```python
from build123d import *

# Parameters (mm, degrees)
SKETCH1_W                                     = 230
SKETCH1_H                                     = 123
SKETCH1_W_2                                   = 206
SKETCH1_H_2                                   = 99
BOSS_EXTRUDE1_DEPTH                           = 5
SKETCH2_W                                     = 230
SKETCH2_H                                     = 5
BOSS_EXTRUDE2_DEPTH                           = 6
BOSS_EXTRUDE3_DEPTH                           = 5
FILLET1_R                                     = 15
BOSS_EXTRUDE4_DEPTH                           = 4
FILLET2_R                                     = 5
FILLET3_R                                     = 3
CSK_FOR_4_FLAT_HEAD_MACHINE_SCREW1_AT_2_COUNT = 2
CSK_FOR_4_FLAT_HEAD_MACHINE_SCREW1_AT_2_PITCH = 30
CSK_FOR_4_FLAT_HEAD_MACHINE_SCREW1_AT_3_COUNT = 2
CSK_FOR_4_FLAT_HEAD_MACHINE_SCREW1_AT_3_PITCH = 225.008888713
CSK_FOR_4_FLAT_HEAD_MACHINE_SCREW1_AT_4_COUNT = 2
CSK_FOR_4_FLAT_HEAD_MACHINE_SCREW1_AT_4_PITCH = 223


with BuildPart() as part:
    # Sketch1 → Boss-Extrude1 (new body)
    with BuildSketch(Plane.XY):
        Rectangle(SKETCH1_W, SKETCH1_H)
        Rectangle(SKETCH1_W_2, SKETCH1_H_2, mode=Mode.SUBTRACT)
    extrude(amount=BOSS_EXTRUDE1_DEPTH)

    # Sketch2 → Boss-Extrude2 (add)
    with BuildSketch(Plane(origin=(0, 61.5, 0), x_dir=(1, 0, 0), z_dir=(0, 1, 0))):
        Polygon((-115, 10), (-115, 0), (115, 0), (115, 10), (115, 93), (105, 93), (105, 10), (-105, 10), (-105, 93), (-115, 93), align=None)
        with Locations((0, -2.5)):
            Rectangle(SKETCH2_W, SKETCH2_H)
    boss_extrude2 = extrude(amount=BOSS_EXTRUDE2_DEPTH)

    # Mirror1: Boss-Extrude2 across plane
    add(boss_extrude2.mirror(Plane.ZX))

    # Sketch3 → Boss-Extrude3 (add)
    with BuildSketch(Plane.ZY.offset(115)):
        Polygon((-93, 61.5), (0, 61.5), (0, -61.5), (-93, -61.5), (-93, -67.5), (5, -67.5), (5, 67.5), (-93, 67.5), align=None)
        Polygon((0, 61.5), (-25, 61.5), (-20, 55.5), (0, 31.5), align=None)
        Polygon((0, -61.5), (0, -31.5), (-20, -55.5), (-25, -61.5), align=None)
        Polygon((-20, 55.5), (-25, 61.5), (-93, 61.5), (-93, 55.5), align=None)
        Polygon((-25, -61.5), (-20, -55.5), (-93, -55.5), (-93, -61.5), align=None)
    boss_extrude3 = extrude(amount=BOSS_EXTRUDE3_DEPTH)

    # Mirror2: Boss-Extrude3 across plane
    add(boss_extrude3.mirror(Plane(origin=(0, 0, 0), x_dir=(0, 0, 1), z_dir=(1, 0, 0))))

    # Fillet1
    fillet1_edges = [part.edges().sort_by_distance(p)[0] for p in [
        (117.5, 55.5, -20),
        (117.5, -55.5, -20),
        (117.5, -31.5, 0),
        (117.5, 31.5, 0),
        (-103, -49.5, 2.5),
        (103, -49.5, 2.5),
        (103, 49.5, 2.5),
        (-103, 49.5, 2.5),
        (105, 64.5, -10),
        (-105, 64.5, -10),
        (-105, -64.5, -10),
        (105, -64.5, -10),
        (-117.5, 55.5, -20),
        (-117.5, 31.5, 0),
        (-117.5, -31.5, 0),
        (-117.5, -55.5, -20),
    ]]
    fillet(fillet1_edges, radius=FILLET1_R)

    # Sketch4 → Boss-Extrude4 (add, symmetric)
    with BuildSketch(Plane(origin=(0, 0, 0), x_dir=(1, 0, 0), z_dir=(0, 1, 0))):
        Polygon((-120, 96.464101615), (-120, 0), (-116.5, 0), (-116.5, 90), (-110.5, 93.464101615), (-110.5, 96.464101615), align=None)
    extrude(amount=BOSS_EXTRUDE4_DEPTH, both=True)

    # Fillet2
    fillet2_edges = [part.edges().sort_by_distance(p)[0] for p in [
        (-118.25, 4, 0),
        (-118.25, -4, 0),
    ]]
    fillet(fillet2_edges, radius=FILLET2_R)

    # Fillet3
    fillet3_edges = [part.edges().sort_by_distance(p)[0] for p in [
        (120, 61.5, -93),
        (120, -61.5, -93),
        (105, 64.5, -93),
        (-120, 0, -96.464101615),
        (-105, 64.5, -93),
        (-105, -64.5, -93),
        (105, -64.5, -93),
        (-120, -61.5, -93),
        (-120, 61.5, -93),
    ]]
    fillet(fillet3_edges, radius=FILLET3_R)

    # Sketch6 → CSK for #4 Flat Head Machine Screw1 (revolve, cut)
    with BuildSketch(Plane(origin=(111.5, 61.5, -68), x_dir=(0, 0, -1), z_dir=(1, 0, 0))):
        Polygon((0, 0), (0, 6), (1.63195, 6), (1.63195, 2.409835609), (2.857501397, 1), (2.857501397, 0), align=None)
    csk_for_4_flat_head_machine_screw1 = revolve(axis=Axis((111.5, 55.15, -68), (0, 1, 0)), mode=Mode.SUBTRACT)

    # CSK for #4 Flat Head Machine Screw1 at 2: CSK for #4 Flat Head Machine Screw1 ×2
    with Locations(*[(0, 0, i * CSK_FOR_4_FLAT_HEAD_MACHINE_SCREW1_AT_2_PITCH) for i in range(1, CSK_FOR_4_FLAT_HEAD_MACHINE_SCREW1_AT_2_COUNT)]):
        add(csk_for_4_flat_head_machine_screw1, mode=Mode.SUBTRACT)

    # CSK for #4 Flat Head Machine Screw1 at 3: CSK for #4 Flat Head Machine Screw1 ×2
    with Locations(*[Vector(-0.991071958, 0, 0.133328066) * (i * CSK_FOR_4_FLAT_HEAD_MACHINE_SCREW1_AT_3_PITCH) for i in range(1, CSK_FOR_4_FLAT_HEAD_MACHINE_SCREW1_AT_3_COUNT)]):
        add(csk_for_4_flat_head_machine_screw1, mode=Mode.SUBTRACT)

    # CSK for #4 Flat Head Machine Screw1 at 4: CSK for #4 Flat Head Machine Screw1 ×2
    with Locations(*[(-i * CSK_FOR_4_FLAT_HEAD_MACHINE_SCREW1_AT_4_PITCH, 0, 0) for i in range(1, CSK_FOR_4_FLAT_HEAD_MACHINE_SCREW1_AT_4_COUNT)]):
        add(csk_for_4_flat_head_machine_screw1, mode=Mode.SUBTRACT)


solid = part.part
```
Can you work these out from the model? Positions are in its coordinate system, mm. A direction names the side the tool comes from. Coordinates: 2 decimals unless noted, no trailing zeros. Loops run counter-clockwise (first coordinate to the right, second up) from the corner with the lowest first, then second, coordinate; pieces in that order, holes last. Notation, with made-up numbers: (36.5, 38) - (48.5, 38) arc R34 cw to (48.5, 75) - close; hole circle Ø7 at (-3.5, 15.25). An arc over 180 degrees is marked (long way). Answer as CSV lines item,"result". Start each with the question number.
1) Suppose I cut it at A-A (z = -79). Please give me the cut outline in (x, y), plus the area to 3 significant figures.
2) I need wall thicknesses on line 1 (Z direction, x = 111.5, y = 61.8); line 2 (Z direction, x = -111, y = 62); line 3 (X direction, y = 62, z = -84). Which ranges of each line are inside material? Lowest first, please. Write a range as from..to.
3) Thinking about a two-plate mould opening in Y: for faces 1 (the flat face through (113, 63, -93)), 2 (the flat face through (117.465, 42.988, -9.574)), 3 (the flat face through (-118, -4, -62)), 4 (the flat face through (8, -67.5, -8)), which applies, pulls with the +Y half, pulls with the -Y half, needs draft (parallel to the pull), parting line crosses it, or undercut?
4) Suppose I cut it at D-D (y = 42.5). Please give me the cut outline in (x, z).
5) Which directions (+Z, -Z, +X, -X, +Y, -Y) give clear straight access to the entire face, cutting with the end or side of a thin tool? Please do faces 5 (the cylindrical face through (-98.72, 44.99, 2.54)), 6 (the flat face through (117.46, -42.79, -9.41)), 7 (the flat face through (115, 57, -36)), 8 (the cylindrical face through (-108.965, 61.993, -69.319)).
6) For pin 1 (1.8 mm diameter, centred on x = 5.5, y = 65, fed in from -Z); pin 2 (1.5 mm diameter, centred on y = -0.5, z = -94.5, fed in from +X); pin 3 (4.5 mm diameter, centred on x = 114.5, y = 58.5, fed in from -Z), each with a flat end and sliding along its axis, tell me the tip position at first contact or that it passes through.
7) Suppose I cut it at B-B (y = -18). Please give me the cut outline in (x, z).
8) Suppose I cut it at C-C (z = -22). Please give me the cut outline in (x, y), plus the area to 3 significant figures.
Check result:
1,outline,"(-120, -67.5) - (-105, -67.5) - (-105, -61.5) - (-115, -61.5) - (-115, -55.5) - (-120, -55.5) - close; (-120, -4) - (-116.5, -4) - (-116.5, 4) - (-120, 4) - close; (-120, 55.5) - (-115, 55.5) - (-115, 61.5) - (-105, 61.5) - (-105, 67.5) - (-120, 67.5) - close; (105, -67.5) - (120, -67.5) - (120, -55.5) - (115, -55.5) - (115, -61.5) - (105, -61.5) - close; (105, 61.5) - (115, 61.5) - (115, 55.5) - (120, 55.5) - (120, 67.5) - (105, 67.5) - close"
1,area,"508 mm²"
2,line 1,"z = -93..-70.86, -65.14..-40.86, -35.14..5"
2,line 2,"z = -93..-70.81, -65.19..-40.81, -35.19..5"
2,line 3,"x = -120..-105, 105..120"
3,face 1,"needs draft"
3,face 2,"undercut"
3,face 3,"undercut"
3,face 4,"pulls with the -Y half"
4,outline,"(-120, -9.17) - (-115, -9.17) - (-115, 0) - (-100.69, 0) - (-100.69, 5) - (-120, 5) - close; (100.69, 0) - (115, 0) - (115, -9.17) - (120, -9.17) - (120, 5) - (100.69, 5) - close"
5,face 5,"+Z, -Z"
5,face 6,"-Z, +X, -X"
5,face 7,"-Z"
5,face 8,"none"
6,pin 1,"stops at z = -10"
6,pin 2,"stops at x = -110.5"
6,pin 3,"stops at z = -93"
7,outline,"(-120, 0) - (-103, 0) - (-103, 5) - (-120, 5) - close; (103, 0) - (120, 0) - (120, 5) - (103, 5) - close"
8,outline,"(-120, -67.5) - (-104.7, -67.5) - (-104.7, -61.5) - (-115, -61.5) - (-115, -54.63) - (-120, -54.63) - close; (-120, -4) - (-116.5, -4) - (-116.5, 4) - (-120, 4) - close; (-120, 54.63) - (-115, 54.63) - (-115, 61.5) - (-104.7, 61.5) - (-104.7, 67.5) - (-120, 67.5) - close; (104.7, -67.5) - (120, -67.5) - (120, -54.63) - (115, -54.63) - (115, -61.5) - (104.7, -61.5) - close; (104.7, 61.5) - (115, 61.5) - (115, 54.63) - (120, 54.63) - (120, 67.5) - (104.7, 67.5) - close"
8,area,"533 mm²"
